The listing builds one solid part. Answer for the finished solid, in the listing's coordinates (mm). A direction names the side the tool comes from. Coordinates: 2 decimals unless noted, no trailing zeros. Loops run counter-clockwise (first coordinate to the right, second up) from the corner with the lowest first, then second, coordinate; pieces in that order, holes last. Notation, with made-up numbers: M -37,12 L 20,12 A36 ccw 20,51 Z; hole C 22.25,24 d9. An arc over 180 degrees is marked long. Answer as a JSON object with one key per item and string values. Group by question number.
1. A cutting plane is placed at D-D on y = -16.25. Give the vertices of the cut face in (x, z), and give its area (3 significant figures).
2. A cutting plane is placed at A-A on x = 12.5. Give the vertices of the cut face in (y, z), and give its area (3 significant figures).
3. Straight lines are drawn through the part: L1, parallel to X at y = -14.25, z = 7.5; L2, parallel to Z at x = 12.5, y = -17; L3, parallel to X at y = -14, z = 4.75. For each, find the intervals that lie inside material, in ascending order.
4. A cutting plane is placed at B-B on y = -10. Give the vertices of the cut face in (x, z).
5. Determine the mould class of faces 3 (the face through (11.979, -6.034, 7.395)), 4 (the face through (12, 0, 7)), 5 (the face through (0, -10, 7)) for opening direction Y: released by +Y, released by -Y, zero draft, split by the parting line, or undercut.
6. Given pin 1 (5 mm diameter, centred on x = 14, z = 9, fed in from -Y), flat-ended and moving along its own axis, determine where the tip first touches the part or whether it passes through.
7. A cutting plane is placed at C-C on z = 7.5. Give the vertices of the cut face in (x, y).
8. For faces 1 (the face through (15.27, -16.37, 6.35)), 2 (the face through (12, -5, 15)), determine the directions among +Z, -Z, +X, -X, +Y, -Y from which every point of the face is accessible in a straight line to the end or side of a thin tool.
from build123d import *

# Parameters (mm, degrees)
F0_W     = 25
F0_H     = 20
F0_R     = 4
F1_DEPTH = 15
F2_R     = 3
F3_DEPTH = 10


with BuildPart() as f1:
    # F0 (on Top) → F1 (new body)
    with BuildSketch(Plane.XY):
        with Locations((12.5, -10)):
            Rectangle(F0_W, F0_H)
        with Locations((12.5, -10)):
            Circle(F0_R, mode=Mode.SUBTRACT)
    extrude(amount=F1_DEPTH)

    # F2 (on face) → F3 (cut)
    with BuildSketch(Plane.XZ.offset(20)):
        with Locations((12.5, 7.5)):
            Circle(F2_R)
    extrude(amount=-F3_DEPTH, mode=Mode.SUBTRACT)


solid = f1.part
From the geometry:
{
 "1": {"outline": "M 0,0 L 25,0 L 25,15 L 0,15 Z; hole C 12.5,7.5 d6", "area": "347 mm²"},
 "2": {"outline": "M -20,0 L -14,0 L -14,4.5 L -20,4.5 Z; M -20,10.5 L -14,10.5 L -14,15 L -20,15 Z; M -6,0 L 0,0 L 0,15 L -6,15 Z", "area": "144 mm²"},
 "3": {"L1": "x = 0 to 9.5, 15.5 to 25", "L2": "z = 0 to 4.5, 10.5 to 15", "L3": "x = 0 to 11.3, 13.7 to 25"},
 "4": {"outline": "M 0,0 L 8.5,0 L 8.5,15 L 0,15 Z; M 16.5,0 L 25,0 L 25,15 L 16.5,15 Z"},
 "5": {"face 3": "undercut", "face 4": "released by +Y", "face 5": "zero draft"},
 "6": {"pin 1": "stops at y = -20"},
 "7": {"outline": "M 0,-20 L 9.5,-20 L 9.5,-12.65 A4 cw long 15.5,-12.65 L 15.5,-20 L 25,-20 L 25,0 L 0,0 Z"},
 "8": {"face 1": "-Y", "face 2": "+Z, +X, -X, +Y, -Y"}
}
